Read the model definition and answer for the solid it produces. Units are mm, in the model's axes. Round coordinates to 2 decimals unless told otherwise and drop trailing zeros. Order: outer loops, then holes, each group sorted by start corner. A loop starts at its lowest first (then second) coordinate and runs counter-clockwise, first axis right, second up. Notation, with made-up numbers: (52, -15) -> (69, -15) arc R19 ccw to (69, 10) -> close; hole circle Ø2 at (53, -15.75). An arc over 180 degrees is marked (long way). Use a Markdown table: item, result. Add a question column.
1. Section A-A, the plane y = 166.75 is taken. Give the vertices of the cut face in (x, z).
2. Given pin 1 (8 mm diameter, centred on x = 37.5, y = 182.5, fed in from -Z); pin 2 (0.8 mm diameter, centred on y = 81, z = 2, fed in from +X); pin 3 (1.6 mm diameter, centred on y = 76.5, z = 2.5, fed in from -X), each flat-ended and moving along its own axis, determine where each tip first touches the part or whether it passes through.
3. Consider L1, parallel to X at y = 195.25, z = 2.4; L2, parallel to Y at x = 24.75, z = 0.85; L3, parallel to X at y = 128.5, z = 2.75. Determine where each line is inside the solid, lowest interval first. Write a range as [from, to].
4. Section B-B, the plane y = 138.25 is taken. Give the number of separate pieces and of enclosed holes in the cut face, then the cut area to 3 significant figures.
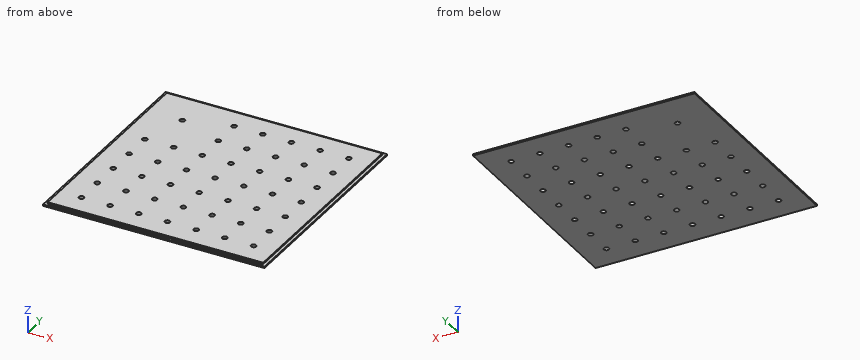
Autodesk Inventor part; units mm, degrees
ref_plane "YZ Plane" through (0, 0, 0) normal (1, 0, 0) x (0, 1, 0)
ref_plane "XZ Plane" through (0, 0, 0) normal (0, 1, 0) x (-1, 0, 0)
ref_plane "XY Plane" through (0, 0, 0) normal (0, 0, 1) x (1, 0, 0)
sketch "Sketch2" plane through (0, 0, 0) normal (0, 0, 1) x (1, 0, 0)
  line L0 (0, 0) -> (220, 0)
  line L1 (220, 0) -> (220, 220)
  line L2 (220, 220) -> (0, 220)
  line L3 (0, 220) -> (0, 0)
  dimension "d0" = 220
  dimension "d1" = 220
extrude "Extrusion1" add sketch "Sketch2" along normal blind 3
sketch "Sketch3" plane through (0, 0, 3) normal (0, 0, 1) x (1, 0, 0)
  line L0 (3, 3) -> (217, 3)
  line L1 (217, 3) -> (217, 217)
  line L2 (217, 217) -> (3, 217)
  line L3 (3, 217) -> (3, 3)
  line L4 (3, 3) -> (217, 217) construction
  line L5 (217, 3) -> (3, 217) construction
  line L6 (0, 220) -> (220, 220)
  line L7 (220, 220) -> (220, 0)
  line L8 (220, 0) -> (0, 0)
  line L9 (0, 0) -> (0, 220)
  point P0 (110, 110)
  dimension "d4" = 214
  dimension "d5" = 214
  dimension "d6" = 220
  dimension "d7" = 220
extrude "Extrusion2" cut sketch "Sketch3" against normal blind 1.5
sketch "Sketch4" plane through (0, 0, 0) normal (0, 0, -1) x (-1, 0, 0)
  line L0 (-210, 10) -> (-10, 10)
  line L1 (-10, 10) -> (-10, 210)
  line L2 (-10, 210) -> (-210, 210)
  line L3 (-210, 210) -> (-210, 10)
  line L4 (-210, 10) -> (-10, 210) construction
  line L5 (-10, 10) -> (-210, 210) construction
  line L6 (-210, 10) -> (-181.5, 10)
  line L7 (-181.5, 10) -> (-181.5, 38.5)
  line L8 (-181.5, 38.5) -> (-210, 38.5)
  line L9 (-210, 38.5) -> (-210, 10)
  circle A0 centre (-195.75, 24.25) radius 2.5
  point P0 (0, 0)
  point P1 (-110, 110)
  dimension "d10" = 200
  dimension "d11" = 200
  dimension "d12" = 28.5
  dimension "d13" = 28.5
  dimension "d14" = 5
extrude "Extrusion3" cut sketch "Sketch4" against normal blind 3 contours A0
pattern_linear "Rectangular Pattern1" count 5 spacing 28.5 along (0, 1, 0) count 7 spacing 28.5 along (-1, 0, 0) of "Extrusion3"
sketch "Sketch5" plane through (0, 0, 0) normal (0, 0, -1) x (-1, 0, 0)
  circle A0 centre (-195.75, 138.25) radius 2.5
  line L0 (-195.75, 138.25) -> (-195.75, 166.75)
  circle A1 centre (-195.75, 166.75) radius 2.5
  point P0 (0, 0)
  dimension "d23" = 28.5
  dimension "d24" = 5
extrude "Extrusion4" cut sketch "Sketch5" against normal blind 3 contours A1
pattern_linear "Rectangular Pattern2" count 5 spacing 28.5 along (-1, 0, 0) count 2 spacing 28.5 along (0, 1, 0) of "Extrusion4"
sketch "Sketch6" plane through (0, 0, 0) normal (0, 0, -1) x (-1, 0, 0)
  line L0 (-10, 10) -> (-210, 10)
  line L1 (-210, 10) -> (-210, 210)
  line L2 (-210, 210) -> (-10, 210)
  line L3 (-10, 210) -> (-10, 10)
  line L4 (-10, 10) -> (-210, 210) construction
  line L5 (-210, 10) -> (-10, 210) construction
  line L6 (-10, 210) -> (-65, 210)
  line L7 (-65, 210) -> (-65, 155)
  line L8 (-65, 155) -> (-10, 155)
  line L9 (-10, 155) -> (-10, 210)
  circle A0 centre (-37.5, 182.5) radius 2.5
  point P0 (0, 0)
  point P1 (-110, 110)
  dimension "d33" = 200
  dimension "d34" = 200
  dimension "d35" = 55
  dimension "d36" = 55
  dimension "d37" = 5
extrude "Extrusion5" cut sketch "Sketch6" against normal blind 3 contours A0
sketch "Sketch7" plane through (0, 0, 0) normal (0, 0, -1) x (-1, 0, 0)
  point P0 (0, 0)
properties part number "inert låg"
Verdict:
| question | item | result |
|---|---|---|
| 1 | outline | (0, 0) -> (79.25, 0) -> (79.25, 3) -> (3, 3) -> (3, 1.5) -> (0, 1.5) -> close; (84.25, 0) -> (107.75, 0) -> (107.75, 3) -> (84.25, 3) -> close; (112.75, 0) -> (136.25, 0) -> (136.25, 3) -> (112.75, 3) -> close; (141.25, 0) -> (164.75, 0) -> (164.75, 3) -> (141.25, 3) -> close; (169.75, 0) -> (193.25, 0) -> (193.25, 3) -> (169.75, 3) -> close; (198.25, 0) -> (220, 0) -> (220, 1.5) -> (217, 1.5) -> (217, 3) -> (198.25, 3) -> close |
| 2 | pin 1 | stops at z = 0 |
| 2 | pin 2 | stops at x = 217 |
| 2 | pin 3 | stops at x = 3 |
| 3 | L1 | x = [3, 79.25], [84.25, 107.75], [112.75, 136.25], [141.25, 164.75], [169.75, 193.25], [198.25, 217] |
| 3 | L2 | y = [0, 21.75], [26.75, 50.25], [55.25, 78.75], [83.75, 107.25], [112.25, 135.75], [140.75, 220] |
| 3 | L3 | x = [3, 217] |
| 4 | separate pieces | 8 |
| 4 | enclosed holes | 0 |
| 4 | area | 546 mm2 |
